Check sheet for the modelled part. Datum: model origin and axes. Units: mm. A direction names the side the tool comes from. Give positions to 0.01 mm unless a question says otherwise; leave off trailing zeros. Order: outer loops, then holes, each group sorted by start corner. A loop starts at its lowest first (then second) coordinate and runs counter-clockwise, first axis right, second up.
```python
from build123d import *

# Parameters (mm, degrees)
BOSS_EXTRUDE1_DEPTH = 3
CHAMFER1_SIZE       = 0.5


with BuildPart() as part:
    # Sketch1 → Boss-Extrude1 (new body)
    with BuildSketch(Plane.XZ):
        Polygon((-2.020725942, 3.5), (-4.041451884, 0), (-2.020725942, -3.5), (2.020725942, -3.5), (4.041451884, 0), (2.020725942, 3.5), align=None)
    extrude(amount=-BOSS_EXTRUDE1_DEPTH)

    # Sketch2 → Revolve1 (revolve)
    with BuildSketch(Plane(origin=(0, 0, 0), x_dir=(-1, 0, 0), z_dir=(0, 0, -1))):
        Polygon((-2.5, 3), (0, 3), (0, 10.5), (-3, 10.5), (-3, 4.5), (-2.5, 4.5), align=None)
    revolve(axis=Axis((0, 3, 0), (0, 1, 0)))

    # Sketch3 → Revolve2 (revolve)
    with BuildSketch(Plane.XY):
        Polygon((2.5, 0), (0, 0), (0, -2), (0.5, -2), align=None)
    revolve(axis=Axis((0, 0, 0), (0, -1, 0)))

    # Sketch4 → Cut-Revolve1 (revolve, cut)
    with BuildSketch(Plane(origin=(0, 0, 0), x_dir=(-1, 0, 0), z_dir=(0, 0, -1))):
        Polygon((-0.15, -2), (0, -2), (0, 10.5), (-1, 10.5), (-1, 0), (-0.75, -0.227272727), (-0.75, -0.7), (-0.15, -1.2), align=None)
    revolve(axis=Axis((0, -2, 0), (0, 1, 0)), mode=Mode.SUBTRACT)

    # Chamfer1
    chamfer1_edges = [part.edges().sort_by_distance(p)[0] for p in [
        (-3, 10.5, 0),
        (-1, 10.5, 0),
    ]]
    chamfer(chamfer1_edges, length=CHAMFER1_SIZE)


solid = part.part
```
(1) Gauge pin test, flat ends, axial feed: pin 1 Ø1.5 at (x, y) = (-1, 4.5) entering from -Z; pin 2 Ø1.5 at (x, z) = (-3, -0.5) entering from -Y; pin 3 Ø1.4 at (x, z) = (0, 0) entering from +Y. Record the tip position at first contact, or that the pin passes through.
Response values:
pin 1: stops at z = -2.99
pin 2: stops at y = -0.21
pin 3: stops at y = -0.74
(2) Cross-section at B-B on y = 3.75. Enter the section's corners in (x, z).
Response values:
outline: circle Ø5 at (0, 0); hole circle Ø2 at (0, 0)
(3) Material ranges on L1, parallel to Z at x = 0, y = 7; L2, parallel to X at y = 3.5, z = 2; L3, parallel to X at y = -0.45, z = 0, recorded low to high.
Response values:
L1: z = -3 to -1, 1 to 3
L2: x = -1.5 to 1.5
L3: x = -2.05 to -0.75, 0.75 to 2.05
(4) Cross-section at D-D on x = 3.75. Enter the section's corners in (y, z), then the cut area to 3 significant figures.
Response values:
outline: (0, -0.5) - (3, -0.5) - (3, 0.5) - (0, 0.5) - close
area: 3.03 mm2
(5) Release check for a two-part mould opening along X. For faces 5 (the face through (0, 1, 3.5)), 6 (the face through (0.391, -1.653, -0.752)), 7 (the face through (-0.75, -0.47, -0.03)) record: released by +X, released by -X, zero draft, split by the parting line, or undercut.
Response values:
face 5: zero draft
face 6: split by the parting line
face 7: undercut
(6) Cross-section at C-C on y = 6.5. Enter the section's corners in (x, z), then the cut area to 3 significant figures.
Response values:
outline: circle Ø6 at (0, 0); hole circle Ø2 at (0, 0)
area: 25.1 mm2
(7) Set-up check for faces 1 (the face through (-3, 1.5, 1.8)), 2 (the face through (3, 0, 0)), 3 (the face through (-0.54, 3.74, 2.44)), 4 (the face through (0, 5, 1)): record each of +Z, -Z, +X, -X, +Y, -Y from which the full face is reachable in a straight line by a thin tool's end or side.
Response values:
face 1: +Z, -X, +Y, -Y
face 2: -Y
face 3: none
face 4: +Y
